Read the model definition and answer for the solid it produces. Units are mm, in the model's axes. Coordinates: 2 decimals unless noted, no trailing zeros. Order: outer loops, then holes, each group sorted by start corner. A loop starts at its lowest first (then second) coordinate and runs counter-clockwise, first axis right, second up.
```python
from build123d import *

# Parameters (mm, degrees)
PAD_DEPTH    = 5
CHAMFER_SIZE = 4


with BuildPart() as part:
    # Sketch → Pad (new body)
    with BuildSketch(Plane.XZ):
        Polygon((-50, -35), (50, -25), (50, 25), (-50, 35), align=None)
    extrude(amount=PAD_DEPTH)

    # Chamfer
    chamfer_edges = [part.edges().sort_by_distance(p)[0] for p in [
        (0, 0, 30),
        (50, 0, 0),
        (0, 0, -30),
        (-50, 0, 0),
    ]]
    chamfer(chamfer_edges, length=CHAMFER_SIZE)


solid = part.part
```
1) A cutting plane is placed at A-A, the plane z = 7.5. Determine the outline of the cut face in (x, y), and give its area (3 significant figures).
A:
outline: (-50, -5) - (50, -5) - (50, -4) - (46, 0) - (-46, 0) - (-50, -4) - close
area: 484 mm2
2) Straight lines are drawn through the part: line 1 (X direction, y = -2.65, z = 22); line 2 (X direction, y = -1.1, z = 13); line 3 (Z direction, x = 4.5, y = -3.6). For each, find the intervals that lie inside material, in ascending order.
A:
line 1: x = -48.65 to 48.65
line 2: x = -47.1 to 47.1
line 3: z = -29.15 to 29.15
3) A cutting plane is placed at B-B, the plane x = -4. Determine the outline of the cut face in (y, z), and give its area (3 significant figures).
A:
outline: (-5, -30.4) - (-4, -30.4) - (0, -26.38) - (0, 26.38) - (-4, 30.4) - (-5, 30.4) - close
area: 288 mm2
4) Flat-ended cylindrical pins translate along their axes: pin 1 Ø1 at (x, y) = (-39, -4.5) entering from +Z; pin 2 Ø3 at (x, y) = (-9.5, -3.5) entering from -Z; pin 3 Ø4 at (x, z) = (25.5, -26) entering from +Y. Find the tip coordinate at first contact, or state that the pin passes through.
A:
pin 1: stops at z = 33.95
pin 2: stops at z = -31.09
pin 3: stops at y = -0.56
